from build123d import *

# Parameters (mm, degrees)
SKETCH1_R               = 23.5
SKETCH1_R_2             = 12.5
BOSS_EXTRUDE1_DEPTH     = 5
SKETCH2_R               = 2
CUT_EXTRUDE1_DEPTH      = 3
SKETCH3_R               = 1.5
CUT_EXTRUDE2_DEPTH      = 90
CUT_EXTRUDE2_DEPTH_BACK = 54
SKETCH6_R               = 4
SKETCH6_R_2             = 1.5
BOSS_EXTRUDE3_DEPTH     = 7
SKETCH7_R               = 4
SKETCH7_R_2             = 1.5
BOSS_EXTRUDE4_DEPTH     = 3


with BuildPart() as part:
    # Sketch1 → Boss-Extrude1 (new body)
    with BuildSketch(Plane.XY):
        Circle(SKETCH1_R)
        Circle(SKETCH1_R_2, mode=Mode.SUBTRACT)
    extrude(amount=BOSS_EXTRUDE1_DEPTH)

    # Sketch2 → Cut-Extrude1 (cut)
    with BuildSketch(Plane.XY.offset(5)):
        with Locations((0, 18)):
            Circle(SKETCH2_R)
        with Locations((15.588457268, -9)):
            Circle(SKETCH2_R)
        with Locations((-15.588457268, -9)):
            Circle(SKETCH2_R)
    extrude(amount=-CUT_EXTRUDE1_DEPTH, mode=Mode.SUBTRACT)

    # Sketch3 → Cut-Extrude2 (cut, two sides)
    with BuildSketch(Plane.XY.offset(5)) as cut_extrude2_sk:
        with Locations((-15.588457268, 9)):
            Circle(SKETCH3_R)
        with Locations((15.588457268, 9)):
            Circle(SKETCH3_R)
        with Locations((0, -18)):
            Circle(SKETCH3_R)
    extrude(amount=CUT_EXTRUDE2_DEPTH, mode=Mode.SUBTRACT)
    extrude(cut_extrude2_sk.sketch, amount=-CUT_EXTRUDE2_DEPTH_BACK, mode=Mode.SUBTRACT)

    # Sketch6 → Boss-Extrude3 (add)
    with BuildSketch(Plane.XY.offset(5)):
        with Locations((-15.588457268, 9)):
            Circle(SKETCH6_R)
        with Locations((-15.588457268, 9)):
            Circle(SKETCH6_R_2, mode=Mode.SUBTRACT)
        with Locations((15.588457268, 9)):
            Circle(SKETCH6_R)
        with Locations((15.588457268, 9)):
            Circle(SKETCH6_R_2, mode=Mode.SUBTRACT)
        with Locations((0, -18)):
            Circle(SKETCH6_R)
        with Locations((0, -18)):
            Circle(SKETCH6_R_2, mode=Mode.SUBTRACT)
    extrude(amount=BOSS_EXTRUDE3_DEPTH)

    # Sketch7 → Boss-Extrude4 (add)
    with BuildSketch(Plane.XY.offset(12)):
        with Locations((-15.588457268, 9)):
            Circle(SKETCH7_R)
        with Locations((-15.588457268, 9)):
            Circle(SKETCH7_R_2, mode=Mode.SUBTRACT)
        with Locations((15.588457268, 9)):
            Circle(SKETCH7_R)
        with Locations((15.588457268, 9)):
            Circle(SKETCH7_R_2, mode=Mode.SUBTRACT)
        with Locations((0, -18)):
            Circle(SKETCH7_R)
        with Locations((0, -18)):
            Circle(SKETCH7_R_2, mode=Mode.SUBTRACT)
    extrude(amount=-BOSS_EXTRUDE4_DEPTH)


solid = part.part
Geometry check sheet. Reference: the model listing, model coordinates, mm. A direction names the side the tool comes from. Coordinates: 2 decimals unless noted, no trailing zeros. Order: outer loops, then holes, each group sorted by start corner. A loop starts at its lowest first (then second) coordinate and runs counter-clockwise, first axis right, second up. Notation, with made-up numbers: (33, 88) - (69, 88) arc R23 ccw to (69, 127) - close; hole circle Ø4 at (65.5, -38.75). An arc over 180 degrees is marked (long way). One line per item, written item: value.
(1) Sectioned sample at C-C (z = 10.5). Enter the section's corners in (x, y).
Data:
outline: circle Ø8 at (-15.59, 9); circle Ø8 at (0, -18); circle Ø8 at (15.59, 9); hole circle Ø3 at (-15.59, 9); hole circle Ø3 at (0, -18); hole circle Ø3 at (15.59, 9)
(2) Sectioned sample at B-B (z = 4). Enter the section's corners in (x, y).
Data:
outline: circle Ø47 at (0, 0); hole circle Ø4 at (-15.59, -9); hole circle Ø3 at (-15.59, 9); hole circle Ø25 at (0, 0); hole circle Ø4 at (0, 18); hole circle Ø3 at (0, -18); hole circle Ø4 at (15.59, -9); hole circle Ø3 at (15.59, 9)
(3) Thickness scan on probe 1 along Y at (x, z) = (0, 3.15); probe 2 along Y at (x, z) = (0, 7.1); probe 3 along Z at (x, y) = (14, -13). Record the ranges inside material, lowest first. Write a range as from..to.
Data:
probe 1: y = -23.5..-19.5, -16.5..-12.5, 12.5..16, 20..23.5
probe 2: y = -22..-19.5, -16.5..-14
probe 3: z = 0..5
(4) Sectioned sample at D-D (y = -6). Enter the section's corners in (x, z).
Data:
outline: (-22.72, 0) - (-10.97, 0) - (-10.97, 5) - (-22.72, 5) - close; (10.97, 0) - (22.72, 0) - (22.72, 5) - (10.97, 5) - close
(5) Depth check by flat-ended pin: pin 1 Ø2 at (y, z) = (-7, 1.5) entering from -X; pin 2 Ø3 at (y, z) = (6.5, 7) entering from -X; pin 3 Ø2.5 at (x, y) = (0, -18) entering from -Z; pin 4 Ø2 at (x, y) = (15, -10) entering from +Z. Enter the tip coordinate at first touch or a pass-through.
Data:
pin 1: stops at x = -22.72
pin 2: stops at x = -19.46
pin 3: passes through
pin 4: stops at z = 5
(6) Sectioned sample at A-A (x = 0). Enter the section's corners in (y, z), and give its area (3 significant figures).
Data:
outline: (-23.5, 0) - (-19.5, 0) - (-19.5, 12) - (-22, 12) - (-22, 5) - (-23.5, 5) - close; (-16.5, 0) - (-12.5, 0) - (-12.5, 5) - (-14, 5) - (-14, 12) - (-16.5, 12) - close; (12.5, 0) - (23.5, 0) - (23.5, 5) - (20, 5) - (20, 2) - (16, 2) - (16, 5) - (12.5, 5) - close
area: 118 mm^2
(7) Release check for a two-part mould opening along X. For faces 3 (the face through (11.923, 3.755, 2.465)), 4 (the face through (10, -10, 0)), 5 (the face through (22.4, 7.1, 2.5)) record: +X half, -X half, draft (parallel to the pull), parting line (faces both ways), or undercut.
Data:
face 3: undercut
face 4: draft
face 5: parting line
(8) Access from +Z, -Z, +X, -X, +Y, -Y to the whole of each face (thin tool, end or side, straight path). Record for faces 1 (the face through (16, 7, 12)), 2 (the face through (0, 20, 4)).
Data:
face 1: +Z, +X, -X, +Y, -Y
face 2: +Z
